Could you check a few things on this model? Use its own coordinates, in mm. Face numbers are marked on the shaded views. A direction names the side the tool comes from. Round coordinates to 2 decimals unless told otherwise and drop trailing zeros. Loops run counter-clockwise (first coordinate to the right, second up) from the corner with the lowest first, then second, coordinate; pieces in that order, holes last. Notation, with made-up numbers: (89, -27.5) - (98, -27.5) arc R17 cw to (98, 4.5) - close; hole circle Ø9 at (66.25, -13). An arc over 180 degrees is marked (long way). Answer as CSV lines item,"result". Start each with the question number.
1) Suppose I cut it at C-C, the plane z = 5. Write out the boundary of the cut face in (x, y).
2) Suppose I cut it at A-A, the plane x = 25.45. Write out the boundary of the cut face in (y, z).
3) Which directions (+Z, -Z, +X, -X, +Y, -Y) give clear straight access to the entire face, cutting with the end or side of a thin tool? Please do the marked faces 1 and 2.
4) Please list where these lines run through material, in increasing order: line 1 along Y through (x, z) = (0.4, 12.5); line 2 along Z through (x, y) = (25.45, 1.15); line 3 along Y through (x, z) = (30, 12.25).
5) Suppose I cut it at D-D, the plane z = 21.5. Write out the boundary of the cut face in (x, y), then the cut area to 3 significant figures.
6) I'm going to push flat-ended pins straight in: pin 1 Ø3 at (y, z) = (14.5, 4) entering from -X; pin 2 Ø5.5 at (y, z) = (6, 12.5) entering from +X; pin 3 Ø5 at (x, z) = (38.5, 10.5) entering from +Y. Where does each tip first touch, or does it pass through?
```python
from build123d import *

# Parameters (mm, degrees)
P_IDAT_VYSUNUT_M1_DEPTH  = 25
SKICA2_R                 = 3.75
SKICA2_R_2               = 1.65
ODEBRAT_VYSUNUT_M2_DEPTH = 25
ZAOBLIT2_R               = 12.5
SKICA3_R                 = 1.65
ODEBRAT_VYSUNUT_M3_DEPTH = 10


with BuildPart() as part:
    # Skica1 → Přidat vysunutím1 (new body)
    with BuildSketch(Plane.XY):
        Polygon((0, 0), (0, 27), (2, 27), (2, 2), (52, 2), (52, 0), align=None)
    extrude(amount=P_IDAT_VYSUNUT_M1_DEPTH)

    # Skica2 → Odebrat vysunutím2 (cut)
    with BuildSketch(Plane.ZY):
        with Locations((12.5, 14.5)):
            Circle(SKICA2_R)
        with Locations((12.5, 23)):
            Circle(SKICA2_R_2)
        with Locations((21, 14.5)):
            Circle(SKICA2_R_2)
        with Locations((4, 14.5)):
            Circle(SKICA2_R_2)
        with Locations((12.5, 6)):
            Circle(SKICA2_R_2)
    extrude(amount=-ODEBRAT_VYSUNUT_M2_DEPTH, mode=Mode.SUBTRACT)

    # Zaoblit2
    zaoblit2_edges = [part.edges().sort_by_distance(p)[0] for p in [
        (1, 27, 0),
        (1, 27, 25),
    ]]
    fillet(zaoblit2_edges, radius=ZAOBLIT2_R - 0.0001)  # a hair under: the kernel refuses the full size

    # Skica3 → Odebrat vysunutím3 (cut)
    with BuildSketch(Plane.XZ):
        with Locations((6.4, 12.5)):
            Circle(SKICA3_R)
        with Locations((25.45, 12.5)):
            Circle(SKICA3_R)
        with Locations((44.5, 12.5)):
            Circle(SKICA3_R)
    extrude(amount=-ODEBRAT_VYSUNUT_M3_DEPTH, mode=Mode.SUBTRACT)


solid = part.part
```
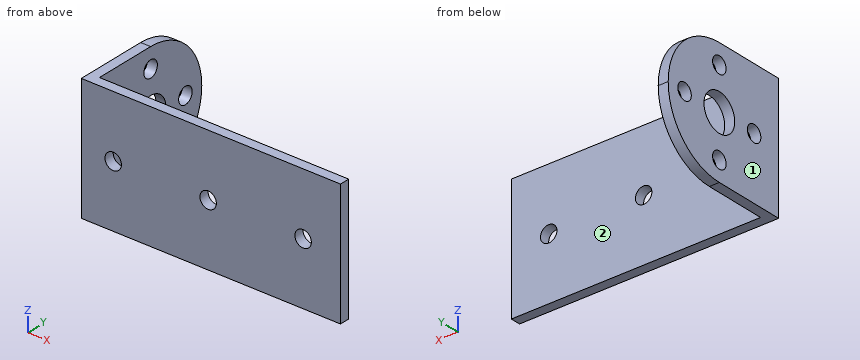
Filled sheet:
1,outline,"(0, 0) - (52, 0) - (52, 2) - (2, 2) - (2, 13.19) - (0, 13.19) - close; (0, 15.81) - (2, 15.81) - (2, 24.5) - (0, 24.5) - close"
2,outline,"(0, 0) - (2, 0) - (2, 10.85) - (0, 10.85) - close; (0, 14.15) - (2, 14.15) - (2, 25) - (0, 25) - close"
3,face 1,"+Z, -Z, -X, +Y, -Y"
3,face 2,"+Z, -Z, +X, +Y"
4,line 1,"0 to 4.35, 7.65 to 10.75, 18.25 to 21.35, 24.65 to 27"
4,line 2,"0 to 10.85, 14.15 to 25"
4,line 3,"0 to 2"
5,outline,"(0, 0) - (52, 0) - (52, 2) - (2, 2) - (2, 12.93) - (0, 12.93) - close; (0, 16.07) - (2, 16.07) - (2, 23.17) - (0, 23.17) - close"
5,area,"140 mm²"
6,pin 1,"through"
6,pin 2,"x = 2"
6,pin 3,"y = 2"
